Autodesk Fusion 360 part; units mm, degrees
sketch "Sketch1" plane through (0, 0, 0) normal (0, 0, 1) x (1, 0, 0)
  line L0 (0, 0) -> (12.7, 0)
  line L1 (12.7, 0) -> (12.7, 12.7)
  line L2 (12.7, 12.7) -> (0, 12.7)
  line L3 (0, 12.7) -> (0, 0)
  circle A0 centre (2.54, 2.54) radius 1.016
  circle A1 centre (10.16, 7.62) radius 1.016
  dimension "d1" = 12.7
  dimension "d2" = 12.7
  dimension "d3" = 2.032
  dimension "d4" = 2.54
  dimension "d5" = 2.54
  dimension "d6" = 2.032
  dimension "d7" = 2.54
  dimension "d8" = 5.08
extrude "Extrude1" add sketch "Sketch1" along normal blind 11.176
Could you check a few things on this model? Use its own coordinates, in mm. Give positions to 0.01 mm unless a question says otherwise; leave off trailing zeros. Order: outer loops, then holes, each group sorted by start corner. A loop starts at its lowest first (then second) coordinate and runs counter-clockwise, first axis right, second up.
1. Suppose I cut it at A-A (y = 2.54). Write out the boundary of the cut face in (x, z).
Answers below:
outline: (0, 0) - (1.52, 0) - (1.52, 11.18) - (0, 11.18) - close; (3.56, 0) - (12.7, 0) - (12.7, 11.18) - (3.56, 11.18) - close
2. Suppose I cut it at C-C (z = 8.5). Write out the boundary of the cut face in (x, y).
Answers below:
outline: (0, 0) - (12.7, 0) - (12.7, 12.7) - (0, 12.7) - close; hole circle Ø2.03 at (2.54, 2.54); hole circle Ø2.03 at (10.16, 7.62)
3. For pin 1 (1.8 mm diameter, centred on x = 10.16, y = 7.62, fed in from -Z), with a flat end and sliding along its axis, tell me the tip position at first contact or that it passes through.
Answers below:
pin 1: passes through
4. Thinking about a two-plate mould opening in Y: for faces 1 (the cylindrical face through (3.086, 1.683, 5.51)), 2 (the flat face through (6, 0, 6)), 3 (the flat face through (6, 6, 0)), which applies, +Y half, -Y half, draft (parallel to the pull), parting line (faces both ways), or undercut?
Answers below:
face 1: undercut
face 2: -Y half
face 3: draft
5. I need wall thicknesses on L1, parallel to Y at x = 2.54, z = 7.5; L2, parallel to Y at x = 10.16, z = 6.5. Which ranges of each line are inside material? Lowest first, please.
Answers below:
L1: y = 0 to 1.52, 3.56 to 12.7
L2: y = 0 to 6.6, 8.64 to 12.7
